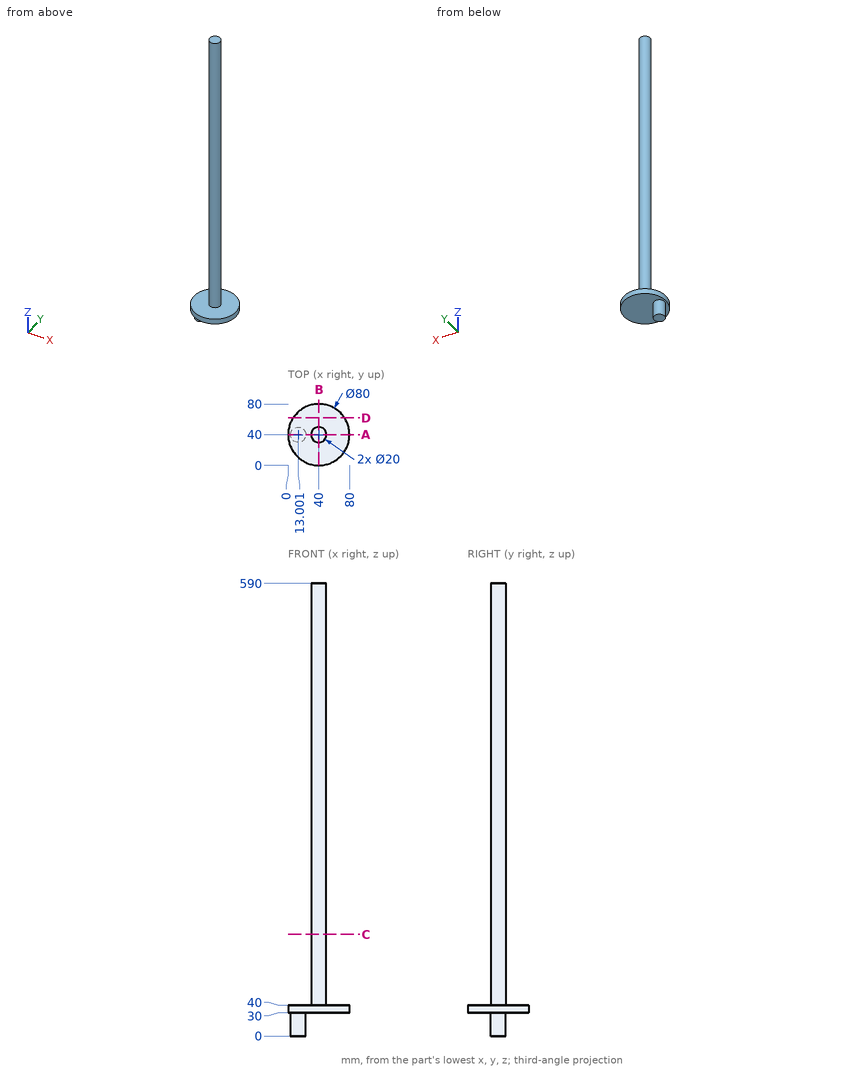
The figure shows three views and two pictorial views of one solid part (mm, origin at its lowest corner). Answer the questions. Round coordinates to 2 decimals unless told otherwise and drop trailing zeros. Write each loop counter-clockwise with the first axis right and the second up, starting at its lowest first coordinate (ties: lowest second). Pieces come first, ordered by that corner, then holes. Notation, with made-up numbers: (57, 17.25) - (88, 17.25) arc R12 cw to (88, 35.25) - close; hole circle Ø1 at (49.5, 76.25). An arc over 180 degrees is marked (long way). Answer in a Markdown table with one row per item. Add a question column.
1. A cutting plane is placed at B-B, the plane x = 40. Determine the outline of the cut face in (y, z).
2. A cutting plane is placed at C-C, the plane z = 132.5. Determine the outline of the cut face in (x, y), and give its area (3 significant figures).
3. A cutting plane is placed at D-D, the plane y = 62. Determine the outline of the cut face in (x, z), and give its area (3 significant figures).
4. A cutting plane is placed at A-A, the plane y = 40. Determine the outline of the cut face in (x, z).
5. Given pin 1 (12 mm diameter, centred on y = 49.5, z = 335, fed in from -X); pin 2 (1.5 mm diameter, centred on x = 68, y = 62.5, fed in from -Z); pin 3 (4 mm diameter, centred on y = 43.5, z = 222, fed in from -X), each flat-ended and moving along its own axis, determine where each tip first touches the part or whether it passes through.
6. Find the intervals of material crossed by line 1 along Y through (x, z) = (39.5, 397); line 2 along Z through (x, y) = (71.5, 51.5); line 3 along Z through (x, y) = (33, 43), in increasing order. Write a range as from..to.
Worked out:
| question | item | result |
|---|---|---|
| 1 | outline | (0, 30) - (80, 30) - (80, 40) - (50, 40) - (50, 590) - (30, 590) - (30, 40) - (0, 40) - close |
| 2 | outline | circle Ø20 at (40, 40) |
| 2 | area | 314 mm^2 |
| 3 | outline | (6.59, 30) - (73.41, 30) - (73.41, 40) - (6.59, 40) - close |
| 3 | area | 668 mm^2 |
| 4 | outline | (0, 30) - (3, 30) - (3, 0) - (23, 0) - (23, 30) - (80, 30) - (80, 40) - (50, 40) - (50, 590) - (30, 590) - (30, 40) - (0, 40) - close |
| 5 | pin 1 | x = 30.63 |
| 5 | pin 2 | z = 30 |
| 5 | pin 3 | x = 30.11 |
| 6 | line 1 | 30.01..49.99 |
| 6 | line 2 | 30..40 |
| 6 | line 3 | 30..590 |
